Answer from the drawing. Dimensions are ordinates in mm from the lowest x, y and z of the part. Coordinates: 2 decimals unless noted, no trailing zeros. Order: outer loops, then holes, each group sorted by start corner. A loop starts at its lowest first (then second) coordinate and runs counter-clockwise, first axis right, second up. Notation, with made-up numbers: (-39, 41) - (-26, 41) arc R28 cw to (-26, 69) - close; hole circle Ø3 at (31, 83.25). An arc over 180 degrees is marked (long way). Use CSV: the item, a comma, the result in double quotes. Start each with the question number.
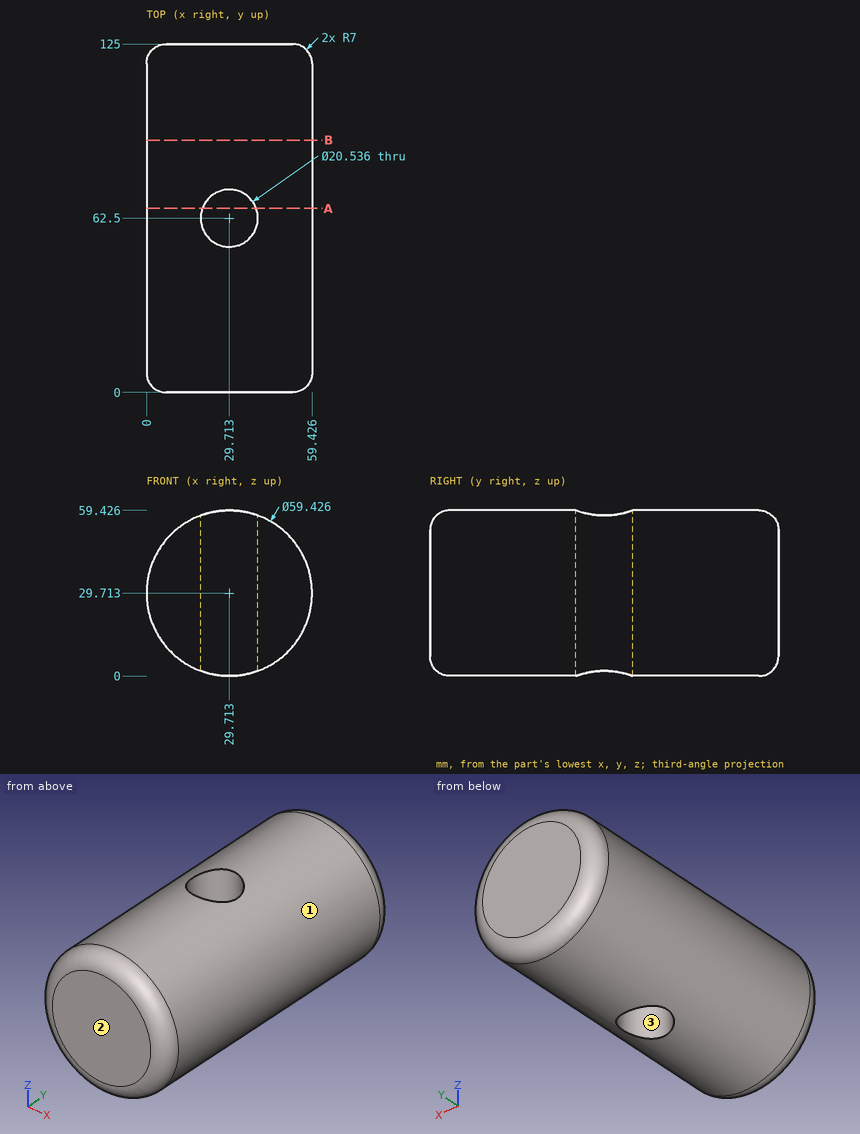
1) For a pull along X with two mould halves and no side action, classify the marked faces 1, 2 and 3 as +X half, -X half, draft (parallel to the pull), parting line (faces both ways), or undercut.
2) Flat-ended cylindrical pins translate along their axes: P1, Ø8, axis at x = 7.5, y = 69.5, coming from the -Z side; P2, Ø2, axis at x = 37, y = 85.5, coming from the -Z side; P3, Ø1, axis at x = 41.5, y = 59.5, coming from the -Z side. Find the tip coordinate at first contact, or state that the pin passes through.
3) The part is cut by section B-B on y = 90.5. Determine the outline of the cut face in (x, z).
4) Straight lines are drawn through the part: line 1 (X direction, y = 62.5, z = 34) (1 decimal); line 2 (X direction, y = 62.5, z = 47.5) (1 decimal); line 3 (X direction, y = 112.5, z = 16). For each, find the intervals that lie inside material, in ascending order. Write a range as [from, to].
5) The part is cut by section A-A on y = 66. Determine the outline of the cut face in (x, z), plus the area to 3 significant figures.
Answer key:
1,face 1,"parting line"
1,face 2,"draft"
1,face 3,"undercut"
2,P1,"z = 6.24"
2,P2,"z = 0.67"
2,P3,"z = 2.23"
3,outline,"circle Ø59.43 at (29.71, 29.71)"
4,line 1,"[0.3, 19.4], [40, 59.1]"
4,line 2,"[5.9, 19.4], [40, 53.5]"
4,line 3,"[3.35, 56.07]"
5,outline,"(20.06, 1.61) - (20.06, 57.81) arc R29.71 ccw to start; (39.37, 1.61) arc R29.71 ccw to (39.37, 57.81) - close"
5,area,"1,650 mm^2"
